```python
from build123d import *

# Parameters (mm, degrees)
SKETCH1_W           = 18
SKETCH1_H           = 14.75
SKETCH1_W_2         = 23
BOSS_EXTRUDE1_DEPTH = 40
CUT_EXTRUDE1_REACH  = 106.057
SKETCH2_R           = 2.6
CUT_EXTRUDE2_REACH  = 106.057
SKETCH3_W           = 10
SKETCH3_H           = 14.75
SKETCH4_W           = 10
SKETCH4_H           = 14.75
CUT_EXTRUDE3_DEPTH  = 102.453449917
CUT_EXTRUDE4_REACH  = 106.057
SKETCH6_R           = 3.25
CHAMFER1_SIZE       = 1
CUT_EXTRUDE5_REACH  = 106.057
SKETCH7_R           = 2.6
SKETCH7_R_2         = 3.1


with BuildPart() as part:
    # Sketch1 → Boss-Extrude1 (new body)
    with BuildSketch(Plane.XY):
        Polygon((0, 0), (0, 63.75), (28, 63.75), (28, 78.05), (56, 78.05), (56, 0), (35, 0), (35, 5), (51, 5), (51, 52.3), (33, 52.3), (33, 38), (5, 38), (5, 5), (19, 5), (19, 0), align=None)
        with Locations((42, 64.675)):
            Rectangle(SKETCH1_W, SKETCH1_H, mode=Mode.SUBTRACT)
        with Locations((16.5, 50.375)):
            Rectangle(SKETCH1_W_2, SKETCH1_H, mode=Mode.SUBTRACT)
    extrude(amount=BOSS_EXTRUDE1_DEPTH)

    # Cut-Extrude1: up to this face of the body (flat: up to its plane)
    cut_extrude1_end = Plane(part.part.faces().sort_by_distance((19, 38, 20))[0])
    # Sketch2 → Cut-Extrude1 (cut, up to the picked face)
    with BuildSketch(Plane(origin=(0, 78.05, 0), x_dir=(1, 0, 0), z_dir=(0, 1, 0)), mode=Mode.PRIVATE) as cut_extrude1_sk1:
        with Locations(Location((19, -15, 0), (0, 0, 270))):
            Circle(SKETCH2_R)
    cut_extrude1_tool1 = split(extrude(cut_extrude1_sk1.sketch, amount=-CUT_EXTRUDE1_REACH, mode=Mode.PRIVATE), bisect_by=cut_extrude1_end, keep=Keep.BOTH, mode=Mode.PRIVATE)
    # Sketch2 → Cut-Extrude1 (cut, up to the picked face)
    with BuildSketch(Plane(origin=(0, 78.05, 0), x_dir=(1, 0, 0), z_dir=(0, 1, 0)), mode=Mode.PRIVATE) as cut_extrude1_sk2:
        with Locations(Location((42, -30, 0), (0, 0, 270))):
            Circle(SKETCH2_R)
    cut_extrude1_tool2 = split(extrude(cut_extrude1_sk2.sketch, amount=-CUT_EXTRUDE1_REACH, mode=Mode.PRIVATE), bisect_by=cut_extrude1_end, keep=Keep.BOTH, mode=Mode.PRIVATE)
    add(cut_extrude1_tool1.solids().sort_by(Axis((19, 78.05, 15), (0, -1, 0)))[0], mode=Mode.SUBTRACT)
    add(cut_extrude1_tool2.solids().sort_by(Axis((42, 78.05, 30), (0, -1, 0)))[0], mode=Mode.SUBTRACT)

    # Sketch3 → Cut-Extrude2 (cut, up to next)
    with BuildSketch(Plane(origin=(56, 0, 0), x_dir=(0, 0, -1), z_dir=(1, 0, 0)), mode=Mode.PRIVATE) as cut_extrude2_sk1:
        with Locations((-25, 64.675)):
            Rectangle(SKETCH3_W, SKETCH3_H)
    cut_extrude2_tool1 = extrude(cut_extrude2_sk1.sketch, amount=-CUT_EXTRUDE2_REACH, mode=Mode.PRIVATE) & part.part
    add(cut_extrude2_tool1.solids().sort_by_distance((56, 64.675, 25))[0], mode=Mode.SUBTRACT)

    # Sketch4 → Cut-Extrude3 (cut, through all)
    with BuildSketch(Plane(origin=(5, 0, 0), x_dir=(0, 0, -1), z_dir=(1, 0, 0))):
        with Locations((-10, 50.375)):
            Rectangle(SKETCH4_W, SKETCH4_H)
    extrude(amount=CUT_EXTRUDE3_DEPTH, mode=Mode.SUBTRACT)

    # Sketch6 → Cut-Extrude4 (cut, up to next)
    with BuildSketch(Plane(origin=(0, 78.05, 0), x_dir=(1, 0, 0), z_dir=(0, 1, 0)), mode=Mode.PRIVATE) as cut_extrude4_sk1:
        with Locations(Location((19, -15, 0), (0, 0, 270))):
            Circle(SKETCH6_R)
    cut_extrude4_tool1 = extrude(cut_extrude4_sk1.sketch, amount=-CUT_EXTRUDE4_REACH, mode=Mode.PRIVATE) & part.part
    # Sketch6 → Cut-Extrude4 (cut, up to next)
    with BuildSketch(Plane(origin=(0, 78.05, 0), x_dir=(1, 0, 0), z_dir=(0, 1, 0)), mode=Mode.PRIVATE) as cut_extrude4_sk2:
        with Locations(Location((42, -30, 0), (0, 0, 270))):
            Circle(SKETCH6_R)
    cut_extrude4_tool2 = extrude(cut_extrude4_sk2.sketch, amount=-CUT_EXTRUDE4_REACH, mode=Mode.PRIVATE) & part.part
    add(cut_extrude4_tool1.solids().sort_by_distance((19, 78.05, 15))[0], mode=Mode.SUBTRACT)
    add(cut_extrude4_tool2.solids().sort_by_distance((42, 78.05, 30))[0], mode=Mode.SUBTRACT)

    # Chamfer1
    chamfer1_edges = [part.edges().sort_by_distance(p)[0] for p in [
        (19, 63.75, 11.75),
        (42, 78.05, 26.75),
    ]]
    chamfer(chamfer1_edges, length=CHAMFER1_SIZE)

    # Sketch7 → Cut-Extrude5 (cut, up to next)
    with BuildSketch(Plane.XZ, mode=Mode.PRIVATE) as cut_extrude5_sk1:
        with Locations((12, 35)):
            Circle(SKETCH7_R)
    cut_extrude5_tool1 = extrude(cut_extrude5_sk1.sketch, amount=-CUT_EXTRUDE5_REACH, mode=Mode.PRIVATE) & part.part
    # Sketch7 → Cut-Extrude5 (cut, up to next)
    with BuildSketch(Plane.XZ, mode=Mode.PRIVATE) as cut_extrude5_sk2:
        with Locations((42, 35)):
            Circle(SKETCH7_R)
    cut_extrude5_tool2 = extrude(cut_extrude5_sk2.sketch, amount=-CUT_EXTRUDE5_REACH, mode=Mode.PRIVATE) & part.part
    # Sketch7 → Cut-Extrude5 (cut, up to next)
    with BuildSketch(Plane.XZ, mode=Mode.PRIVATE) as cut_extrude5_sk3:
        with Locations((12, 15)):
            Circle(SKETCH7_R_2)
    cut_extrude5_tool3 = extrude(cut_extrude5_sk3.sketch, amount=-CUT_EXTRUDE5_REACH, mode=Mode.PRIVATE) & part.part
    # Sketch7 → Cut-Extrude5 (cut, up to next)
    with BuildSketch(Plane.XZ, mode=Mode.PRIVATE) as cut_extrude5_sk4:
        with Locations((42, 15)):
            Circle(SKETCH7_R_2)
    cut_extrude5_tool4 = extrude(cut_extrude5_sk4.sketch, amount=-CUT_EXTRUDE5_REACH, mode=Mode.PRIVATE) & part.part
    add(cut_extrude5_tool1.solids().sort_by_distance((12, 0, 35))[0], mode=Mode.SUBTRACT)
    add(cut_extrude5_tool2.solids().sort_by_distance((42, 0, 35))[0], mode=Mode.SUBTRACT)
    add(cut_extrude5_tool3.solids().sort_by_distance((12, 0, 15))[0], mode=Mode.SUBTRACT)
    add(cut_extrude5_tool4.solids().sort_by_distance((42, 0, 15))[0], mode=Mode.SUBTRACT)


solid = part.part
```
CAD build for the part. Positions are in the model's coordinates, mm. A direction names the side the tool comes from. Coordinates: 2 decimals unless noted, no trailing zeros. Order: outer loops, then holes, each group sorted by start corner. A loop starts at its lowest first (then second) coordinate and runs counter-clockwise, first axis right, second up. Notation, with made-up numbers: (-24, 20) - (-10, 20) arc R14 cw to (-10, 29) - close; hole circle Ø5 at (89, 8.5). An arc over 180 degrees is marked (long way). Use a Markdown table: item, result. Add a question column.
(1) Saw through at D-D (y = 71). Give the cut face in (x, z).
(2) Saw through at A-A (x = 26.5). Give the cut face in (y, z), then the cut area to 3 significant figures.
(3) Flat gauge pins, fed straight in: pin 1 (1 mm diameter, centred on x = 29, z = 29.5, fed in from -Y); pin 2 (7.5 mm diameter, centred on x = 19, z = 15, fed in from +Y); pin 3 (5 mm diameter, centred on x = 11, z = 16, fed in from +Y). Where does each tip first touch, or does it go through?
(4) Which spindle directions (+Z, -Z, +X, -X, +Y, -Y) get a long thin tool onto all of the face, cutting with end or side? Do faces 4 (the face through (44.864, 2.465, 13.813)), 5 (the face through (54, 65, 20)), 6 (the face through (14, 63.75, 20)). Say none if no direction does.
(5) Pull direction Z, two halves, no side cores. Call faces 1 (the face through (28, 40, 40)), 2 (the face through (39.46, 54.83, 29.44)), 3 (the face through (28, 50, 2)): +Z half, -Z half, draft (parallel to the pull), parting line (faces both ways), or undercut.
(6) Drill centre lines: line 1 along Y through (x, z) = (43, 20); line 2 along X through (y, z) = (40.9, 15); line 3 along Z through (x, y) = (42, 2.7). Where is each one in solid material? Low to high. Write a range as [from, to].
(7) Saw through at B-B (y = 35). Give the cut face in (x, z), then the cut area to 3 significant figures.
(8) Saw through at C-C (z = 24). Give the cut face in (x, y).
Solved:
| question | item | result |
|---|---|---|
| 1 | outline | (28, 0) - (33, 0) - (33, 40) - (28, 40) - close; (51, 0) - (56, 0) - (56, 20) - (51, 20) - close; (51, 30) - (56, 30) - (56, 40) - (51, 40) - close |
| 2 | outline | (38, 0) - (43, 0) - (43, 40) - (38, 40) - close; (57.75, 0) - (63.75, 0) - (63.75, 40) - (57.75, 40) - close |
| 2 | area | 440 mm² |
| 3 | pin 1 | stops at y = 38 |
| 3 | pin 2 | stops at y = 63.25 |
| 3 | pin 3 | stops at y = 63.75 |
| 4 | face 4 | -Y |
| 4 | face 5 | +X |
| 4 | face 6 | +Z, -Z, -X, +Y |
| 5 | face 1 | +Z half |
| 5 | face 2 | undercut |
| 5 | face 3 | draft |
| 6 | line 1 | y = [0, 5], [52.3, 57.3], [72.05, 78.05] |
| 6 | line 2 | x = [0, 16.4], [21.6, 33], [51, 56] |
| 6 | line 3 | z = [0, 11.9], [18.1, 32.4], [37.6, 40] |
| 7 | outline | (0, 0) - (5, 0) - (5, 40) - (0, 40) - close; (51, 0) - (56, 0) - (56, 40) - (51, 40) - close |
| 7 | area | 400 mm² |
| 8 | outline | (0, 0) - (19, 0) - (19, 5) - (5, 5) - (5, 38) - (33, 38) - (33, 52.3) - (51, 52.3) - (51, 5) - (35, 5) - (35, 0) - (56, 0) - (56, 57.3) - (33, 57.3) - (33, 72.05) - (56, 72.05) - (56, 78.05) - (28, 78.05) - (28, 63.75) - (0, 63.75) - close; hole (5, 43) - (28, 43) - (28, 57.75) - (5, 57.75) - close |
